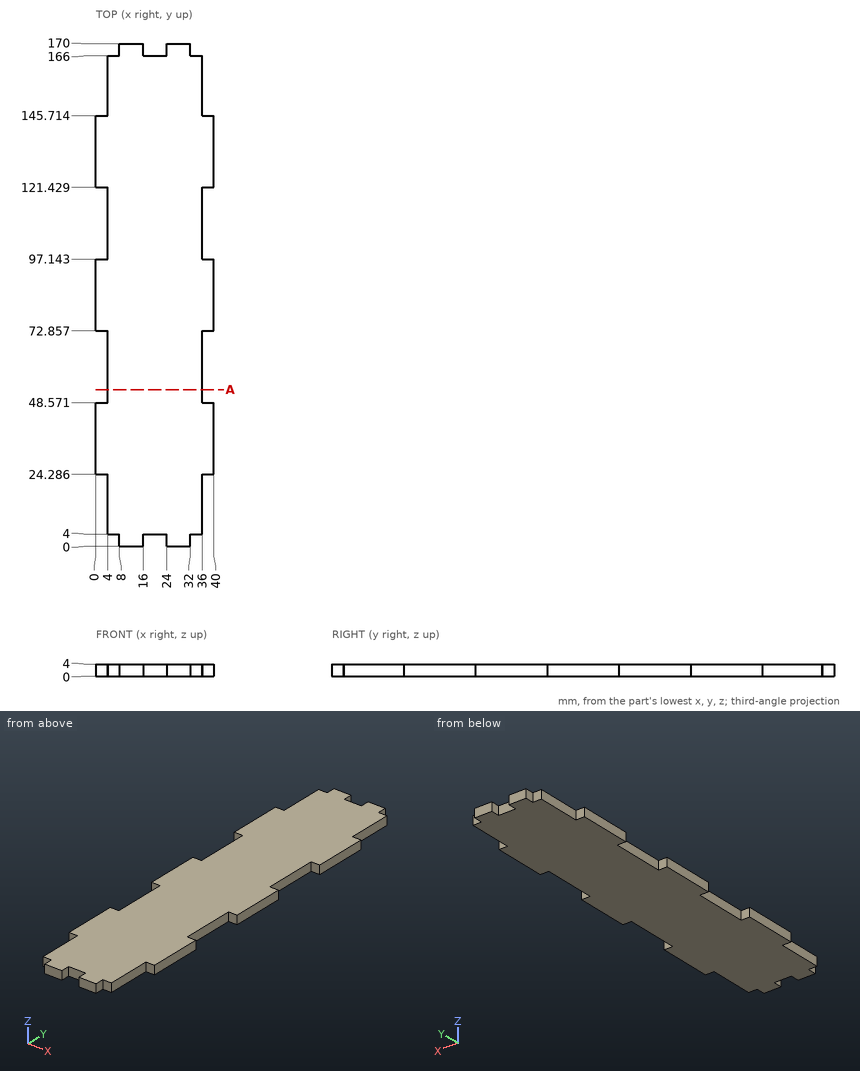
Geometry: see drawing. Coordinates: mm, zero at the bounding-box minimum. Round coordinates to 2 decimals unless told otherwise and drop trailing zeros. Write each loop counter-clockwise with the first axis right and the second up, starting at its lowest first coordinate (ties: lowest second). Pieces come first, ordered by that corner, then holes. Notation, with made-up numbers: (-36.5, 52) - (-1.5, 52) arc R17 ccw to (-1.5, 82) - close; hole circle Ø9 at (-22, -10). An arc over 180 degrees is marked (long way). Use CSV: the item, a comma, the result in double quotes. Start each with the question number.
(1) Material intervals for probe 1 along Y at (x, z) = (38, 0.2) (1 decimal); probe 2 along Y at (x, z) = (20, 2.85); probe 3 along X at (y, z) = (152.5, 0.8), sorted ascending. Write a range as [from, to].
(2) Cut plane A-A, the plane y = 53. Return loops of the section in (x, z), and give its area (3 significant figures).
(3) First-contact query: pin 1 Ø1.2 at (y, z) = (12, 2.5) entering from -X; pin 2 Ø1.2 at (x, z) = (37.5, 2) entering from -Y; pin 3 Ø1.2 at (y, z) = (1.5, 2.5) entering from -X. Flat tips, straight axial feed; report the tip coordinate or a pass-through.
Geometry says:
1,probe 1,"[24.3, 48.6], [72.9, 97.1], [121.4, 145.7]"
1,probe 2,"[4, 166]"
1,probe 3,"[4, 36]"
2,outline,"(4, 0) - (36, 0) - (36, 4) - (4, 4) - close"
2,area,"128 mm²"
3,pin 1,"x = 4"
3,pin 2,"y = 24.29"
3,pin 3,"x = 8"
